Can you work these out from the model? Positions are in its coordinate system, mm. A direction names the side the tool comes from. Coordinates: 2 decimals unless noted, no trailing zeros. Order: outer loops, then holes, each group sorted by start corner. A loop starts at its lowest first (then second) coordinate and runs counter-clockwise, first axis right, second up. Notation, with made-up numbers: (79, 37) -> (103, 37) arc R19 cw to (103, 51) -> close; hole circle Ø3 at (21.5, 39). An arc over 180 degrees is marked (long way). Write item = value, one per line.
```python
from build123d import *

# Parameters (mm, degrees)
SKETCH_W        = 22.5
SKETCH_H        = 66
PAD_DEPTH       = 15
SKETCH001_W     = 12.5
SKETCH001_H     = 75
SKETCH001_W_2   = 4.6
SKETCH001_H_2   = 4.6
POCKET_DEPTH    = 10
SKETCH002_W     = 7
SKETCH002_H     = 7
POCKET001_DEPTH = 5.8
SKETCH004_W     = 1.1
SKETCH004_H     = 4
POCKET002_DEPTH = 10
SKETCH005_W     = 4
SKETCH005_H     = 1.3
POCKET003_DEPTH = 10
SKETCH007_W     = 19.75
SKETCH007_H     = 26.5
POCKET004_DEPTH = 20


with BuildPart() as part:
    # Sketch → Pad (new body)
    with BuildSketch(Plane.XY):
        with Locations((51.75, -67)):
            Rectangle(SKETCH_W, SKETCH_H)
    extrude(amount=PAD_DEPTH)

    # Sketch001 (on DatumPlane) → Pocket (cut)
    with BuildSketch(Plane.XY.offset(15)):
        with Locations((51.75, -57.5)):
            Rectangle(SKETCH001_W, SKETCH001_H)
        with Locations((51.75, -64)):
            Rectangle(SKETCH001_W_2, SKETCH001_H_2, mode=Mode.SUBTRACT)
    extrude(amount=-POCKET_DEPTH, mode=Mode.SUBTRACT)

    # Sketch002 (on DatumPlane) → Pocket001 (cut)
    with BuildSketch(Plane.XY.offset(15)):
        with Locations((51.5, -63.5)):
            Rectangle(SKETCH002_W, SKETCH002_H)
    extrude(amount=-POCKET001_DEPTH, mode=Mode.SUBTRACT)

    # Sketch004 (on DatumPlane) → Pocket002 (cut)
    with BuildSketch(Plane.XY.offset(15)):
        with Locations((51.75, -64)):
            Rectangle(SKETCH004_W, SKETCH004_H)
    extrude(amount=-POCKET002_DEPTH, mode=Mode.SUBTRACT)

    # Sketch005 (on DatumPlane) → Pocket003 (cut)
    with BuildSketch(Plane.XY.offset(15)):
        with Locations((51.75, -64)):
            Rectangle(SKETCH005_W, SKETCH005_H)
    extrude(amount=-POCKET003_DEPTH, mode=Mode.SUBTRACT)

    # Sketch007 (on DatumPlane) → Pocket004 (cut)
    with BuildSketch(Plane.XY.offset(15)):
        with Locations((66.125, -42.25)):
            Rectangle(SKETCH007_W, SKETCH007_H)
    extrude(amount=-POCKET004_DEPTH, mode=Mode.SUBTRACT)


solid = part.part
```
Item 1: If we mould it in two halves opening along Y, with no side actions, what happens to faces 1 (the flat face through (52, -100, 7)), 2 (the flat face through (40.5, -67, 7)), 3 (the flat face through (50, -63.35, 7))? For each: pulls with the +Y half, pulls with the -Y half, needs draft (parallel to the pull), parting line crosses it, or undercut.
A:
face_1 = pulls with the -Y half
face_2 = needs draft
face_3 = undercut
Item 2: I want a section at C-C, the plane x = 48.75. Please give me the cut outline in (y, z), plus the area to 3 significant figures.
A:
outline = (-100, 0) -> (-34, 0) -> (-34, 5) -> (-95, 5) -> (-95, 15) -> (-100, 15) -> close
area = 380 mm2
Item 3: If I drill on probe 1 along X at (y, z) = (-83, 9.75); probe 2 along Y at (x, z) = (50.5, 7.25); probe 3 along Z at (x, y) = (48.75, -67), over which ranges is the centre line in solid material (lowest first)?
A:
probe_1 = 40.5 to 45.5, 58 to 63
probe_2 = -100 to -95, -66.3 to -64.65, -63.35 to -61.7
probe_3 = 0 to 5
Item 4: For faces 4 (the flat face through (49.75, -64, 7)), 5 (the flat face through (60, -55.5, 8)), 6 (the flat face through (53, -65, 9.2)), which set-ups out of +Z, -Z, +X, -X, +Y, -Y let a thin tool reach every point of the face, with its end or its side?
A:
face_4 = +Z
face_5 = +Z, -Z, +X, +Y
face_6 = +Z, +Y
Item 5: I want a section at A-A, the plane y = -78. Please give me the cut outline in (x, z), plus the area to 4 significant figures.
A:
outline = (40.5, 0) -> (63, 0) -> (63, 15) -> (58, 15) -> (58, 5) -> (45.5, 5) -> (45.5, 15) -> (40.5, 15) -> close
area = 212.5 mm2
Item 6: I want a section at B-B, the plane z = 11.25. Please give me the cut outline in (x, y), plus the area to 3 significant figures.
A:
outline = (40.5, -100) -> (63, -100) -> (63, -55.5) -> (58, -55.5) -> (58, -95) -> (45.5, -95) -> (45.5, -34) -> (40.5, -34) -> close
area = 615 mm2
Item 7: I'm going to push flat-ended pins straight in: P1, Ø1.3, axis at x = 52, z = 6.5, coming from the +Y side; P2, Ø2, axis at x = 53.5, z = 11.5, coming from the +Y side; P3, Ø4, axis at y = -39.5, z = 3.5, coming from the +X side. Where does each tip first touch, or does it pass through?
A:
P1 = -61.7
P2 = -95
P3 = 56.25
Item 8: I want a section at D-D, the plane y = -53. Please give me the cut outline in (x, z), plus the area to 3 significant figures.
A:
outline = (40.5, 0) -> (56.25, 0) -> (56.25, 5) -> (45.5, 5) -> (45.5, 15) -> (40.5, 15) -> close
area = 129 mm2
